from build123d import *

# Parameters (mm, degrees)
SKETCH007_W            = 70
SKETCH007_H            = 50
SKETCH007_R            = 7.475
SKETCH007_R_2          = 5.25
PAD010_DEPTH           = 15
POCKET_DEPTH           = 50.001
SKETCH009_W            = 5
SKETCH009_H            = 10
POCKET001_DEPTH        = 15.001
LINEARPATTERN_COUNT    = 2
LINEARPATTERN_PITCH    = 40
SKETCH010_W            = 10
SKETCH010_H            = 5
POCKET002_DEPTH        = 5
LINEARPATTERN001_COUNT = 2
LINEARPATTERN001_PITCH = 35


with BuildPart() as part:
    # Sketch007 → Pad010 (new body)
    with BuildSketch(Plane.XZ):
        with Locations((8.6, 25)):
            Rectangle(SKETCH007_W, SKETCH007_H)
        with Locations((26.05, 29.15)):
            Circle(SKETCH007_R, mode=Mode.SUBTRACT)
        with Locations((-8.85, 29.15)):
            Circle(SKETCH007_R_2, mode=Mode.SUBTRACT)
    extrude(amount=PAD010_DEPTH)

    # Sketch008 (on Face1 of Pad010) → Pocket (cut, through all)
    with BuildSketch(Plane(origin=(0, 0, 50), x_dir=(-1, 0, 0), z_dir=(0, 0, 1))):
        Polygon((-3.6, 15), (-8.6, 10), (-13.6, 15), align=None)
    extrude(amount=-POCKET_DEPTH, mode=Mode.SUBTRACT)

    # Sketch009 (on Face7 of Pocket) → Pocket001 (cut, through all)
    with BuildSketch(Plane.XZ.offset(15)):
        with Locations((16.1, 5)):
            Rectangle(SKETCH009_W, SKETCH009_H)
        with Locations((1.1, 5)):
            Rectangle(SKETCH009_W, SKETCH009_H)
    pocket001 = extrude(amount=-POCKET001_DEPTH, mode=Mode.SUBTRACT)

    # LinearPattern: Pocket001 ×2
    with Locations(*[(0, 0, i * LINEARPATTERN_PITCH) for i in range(1, LINEARPATTERN_COUNT)]):
        add(pocket001, mode=Mode.SUBTRACT)

    # Sketch010 (on Face4 of LinearPattern) → Pocket002 (cut)
    with BuildSketch(Plane.XZ.offset(15)):
        with Locations((8.6, 42.5)):
            Rectangle(SKETCH010_W, SKETCH010_H)
    pocket002 = extrude(amount=-POCKET002_DEPTH, mode=Mode.SUBTRACT)

    # LinearPattern001: Pocket002 ×2
    with Locations(*[(0, 0, -i * LINEARPATTERN001_PITCH) for i in range(1, LINEARPATTERN001_COUNT)]):
        add(pocket002, mode=Mode.SUBTRACT)


with BuildPart() as part_1:
    # Body001 placement: moved
    add(part.part.moved(Location((0, -35, 0))))


solid = part_1.part
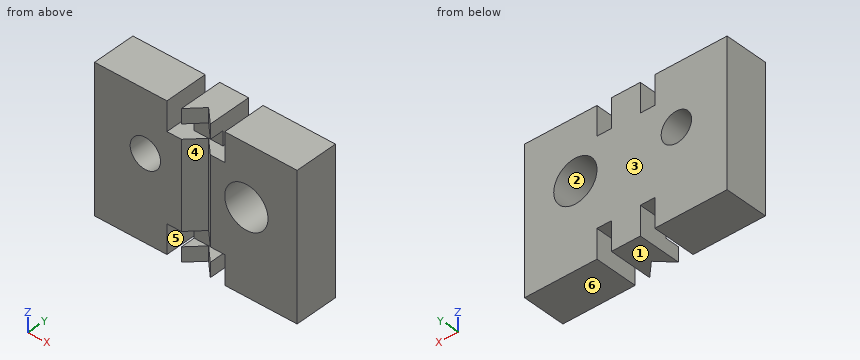
Design review of the part built by this model. Coordinates are the model's own, in mm. Face numbers are marked on the shaded views. A direction names the side the tool comes from. Round coordinates to 2 decimals unless told otherwise and drop trailing zeros. Order: outer loops, then holes, each group sorted by start corner. A loop starts at its lowest first (then second) coordinate and runs counter-clockwise, first axis right, second up.
1) Consider section A-A (y = -46.75). Count the separate pieces of the cut face and the enclosed holes in it, plus the area to 3 significant figures.
The answers:
separate pieces: 6
enclosed holes: 2
area: 2,800 mm2
2) Consider section C-C (z = 29.15). State the section outline as (x, y) points (3 decimals), plus the area to 3 significant figures.
The answers:
outline: (-26.4, -50) - (-14.1, -50) - (-14.1, -35) - (-26.4, -35) - close; (-3.6, -50) - (3.6, -50) - (8.6, -45) - (13.6, -50) - (18.575, -50) - (18.575, -35) - (-3.6, -35) - close; (33.525, -50) - (43.6, -50) - (43.6, -35) - (33.525, -35) - close
area: 643 mm2
3) For L1, parallel to X at y = -44, z = 43; L2, parallel to Z at x = 26.05, y = -42.5 (3 decimals); L3, parallel to Z at x = -8.85, y = -42.5, list the stretches that pass through material, from the lowest coordinate up.
The answers:
L1: x = -26.4 to -1.4, 3.6 to 13.6, 18.6 to 43.6
L2: z = 0 to 21.675, 36.625 to 50
L3: z = 0 to 23.9, 34.4 to 50
4) Consider section D-D (y = -39.5). State the section outline as (x, z) points (3 decimals), plus the area to 3 significant figures.
The answers:
outline: (-26.4, 0) - (-1.4, 0) - (-1.4, 10) - (3.6, 10) - (3.6, 0) - (13.6, 0) - (13.6, 10) - (18.6, 10) - (18.6, 0) - (43.6, 0) - (43.6, 50) - (18.6, 50) - (18.6, 40) - (13.6, 40) - (13.6, 50) - (3.6, 50) - (3.6, 40) - (-1.4, 40) - (-1.4, 50) - (-26.4, 50) - close; hole circle Ø10.5 at (-8.85, 29.15); hole circle Ø14.95 at (26.05, 29.15)
area: 3,040 mm2
5) Consider section B-B (x = 26.05). State the section outline as (y, z) points (3 decimals).
The answers:
outline: (-50, 0) - (-35, 0) - (-35, 21.675) - (-50, 21.675) - close; (-50, 36.625) - (-35, 36.625) - (-35, 50) - (-50, 50) - close
6) Machinability: for the marked faces 4, 5 and 6, which of the approach directions +Z, -Z, +X, -X, +Y, -Y give a long, thin tool a straight path to every point of the face, cutting with its end or side? Answer none if there is none.
The answers:
face 4: +Z, -Z, -Y
face 5: -Z, +Y, -Y
face 6: -Z, +X, -X, +Y, -Y
7) Draft analysis for pull direction Z (two halves, no side actions). For the marked faces 1, 2 and 3, state which applies: released by +Z, released by -Z, zero draft, split by the parting line, or undercut.
The answers:
face 1: released by -Z
face 2: undercut
face 3: zero draft
8) Clearance check with flat-ended pins moving along their axes: pin 1 Ø1.5 at (x, y) = (6.5, -47.5) entering from -Z; pin 2 Ø3 at (x, y) = (1, -41) entering from -Z; pin 3 Ø5.5 at (x, z) = (10.5, 8.5) entering from -Y; pin 4 Ø4 at (x, z) = (9, 41.5) entering from -Y. State where each tip first meets the part, or that it passes through.
The answers:
pin 1: stops at z = 0
pin 2: stops at z = 10
pin 3: stops at y = -49.2
pin 4: stops at y = -46.72
